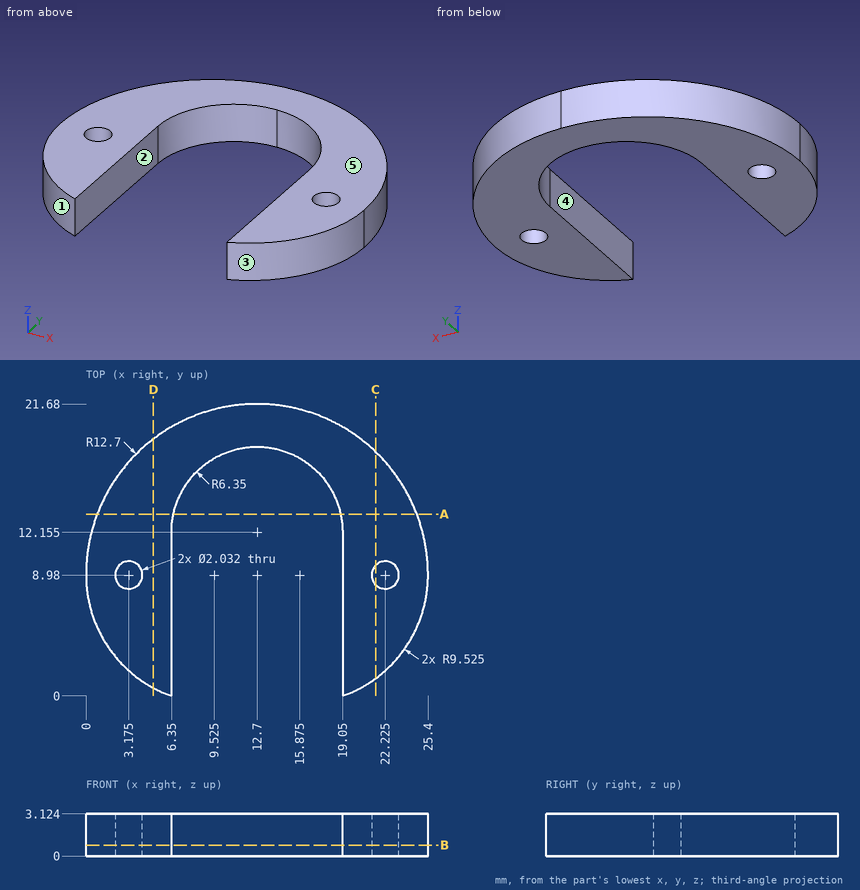
Study the drawing (mm; zero at the part's minimum x, y, z) and answer. A direction names the side the tool comes from. Coordinates: 2 decimals unless noted, no trailing zeros. Write each loop counter-clockwise with the first axis right and the second up, starting at its lowest first coordinate (ties: lowest second). Pieces come first, ordered by that corner, then holes.
Q1. Each of these flat-tipped pins is pushed along its axis until it touches: pin 1 Ø1.5 at (y, z) = (14.5, 1.5) entering from -X; pin 2 Ø1 at (x, z) = (16, 1.5) entering from +Y. Where does it stop, or does it pass through?
Q2. Which of the six approach directions +Z, -Z, +X, -X, +Y, -Y give full straight-line access (tool end or side, diameter ignored) to the marked faces 1 and 2?
Q3. A cutting plane is placed at D-D, the plane x = 5. Give the vertices of the cut face in (y, z).
Q4. A cutting plane is placed at A-A, the plane y = 13.5. Give the vertices of the cut face in (x, z).
Q5. A cutting plane is placed at C-C, the plane x = 21.5. Give the vertices of the cut face in (y, z).
Q6. Determine the mould class of the marked faces 3, 4 and 5 for opening direction X: released by +X, released by -X, zero draft, split by the parting line, or undercut.
Q7. A cutting plane is placed at B-B, the plane z = 0.8. State how many separate pieces and enclosed holes the cut face has, then the cut area to 3 significant figures.
Q8. Find the intervals of material crossed by line 1 (X direction, y = 14.75, z = 2) (1 decimal); line 2 (X direction, y = 10.75, z = 2.7); line 3 (Y direction, x = 2.5, z = 0.65) (1 decimal), in increasing order.
Findings below:
1. pin 1: stops at x = 0.93
1. pin 2: stops at y = 21.37
2. face 1: +Z, -Z, -X, -Y
2. face 2: +Z, -Z, -Y
3. outline: (0.6, 0) - (19.08, 0) - (19.08, 3.12) - (0.6, 3.12) - close
4. outline: (0.83, 0) - (6.49, 0) - (6.49, 3.12) - (0.83, 3.12) - close; (18.91, 0) - (24.57, 0) - (24.57, 3.12) - (18.91, 3.12) - close
5. outline: (1.29, 0) - (8.27, 0) - (8.27, 3.12) - (1.29, 3.12) - close; (9.69, 0) - (18.14, 0) - (18.14, 3.12) - (9.69, 3.12) - close
6. face 3: released by +X
6. face 4: undercut
6. face 5: zero draft
7. separate pieces: 1
7. enclosed holes: 2
7. area: 226 mm2
8. line 1: x = 1.4 to 6.9, 18.5 to 24
8. line 2: x = 0.12 to 6.35, 19.05 to 25.28
8. line 3: y = 2.5 to 8.2, 9.7 to 16.5
